from build123d import *

# Parameters (mm, degrees)
SKETCH1_R               = 10
BOSS_EXTRUDE1_DEPTH     = 15
BOSS_EXTRUDE2_START     = -2
BOSS_EXTRUDE2_OUTLINE_R = 1
BOSS_EXTRUDE2_DEPTH     = 2
SKETCH3_W               = 10
SKETCH3_H               = 3
BOSS_EXTRUDE3_DEPTH     = 2
SKETCH4_W               = 9.5
SKETCH4_H               = 2.5
SKETCH4_R               = 0.25
CUT_EXTRUDE1_DEPTH      = 3
SKETCH5_R               = 1.5
CUT_EXTRUDE2_DEPTH      = 3


# Read off the part's stored shape, not the designer's step: Boss-Extrude2
with BuildPart() as part:
    # Sketch1 → Boss-Extrude1 (new body)
    with BuildSketch(Plane.XY):
        Circle(SKETCH1_R)
    extrude(amount=BOSS_EXTRUDE1_DEPTH)

    # Boss-Extrude2 outline → Boss-Extrude2 (add)
    # profile 1 of 2: a face of its own
    with BuildSketch(Plane(origin=(0, 0, 0), x_dir=(-1, 0, 0), z_dir=(0, 0, -1)).offset(BOSS_EXTRUDE2_START)):
        with BuildLine():
            Line((5.599999975, -8.284926088), (14.179999754, -2.485477473))
            ThreePointArc((14.179999754, -2.485477473), (15.499999574, 0), (14.179999754, 2.485477473))
            Line((14.179999754, 2.485477473), (5.599999975, 8.284926088))
            ThreePointArc((5.599999975, 8.284926088), (10, 0), (5.599999975, -8.284926088))
        make_face()
        with Locations((12.5, 0)):
            Circle(BOSS_EXTRUDE2_OUTLINE_R, mode=Mode.SUBTRACT)
    # profile 2 of 2: a face of its own
    with BuildSketch(Plane(origin=(0, 0, 0), x_dir=(-1, 0, 0), z_dir=(0, 0, -1)).offset(BOSS_EXTRUDE2_START)):
        with BuildLine():
            Line((-14.179999754, -2.485477473), (-5.599999975, -8.284926088))
            ThreePointArc((-5.599999975, -8.284926088), (-10, 0), (-5.599999975, 8.284926088))
            Line((-5.599999975, 8.284926088), (-14.179999754, 2.485477473))
            ThreePointArc((-14.179999754, 2.485477473), (-15.499999574, 0), (-14.179999754, -2.485477473))
        make_face()
        with Locations((-12.5, 0)):
            Circle(BOSS_EXTRUDE2_OUTLINE_R, mode=Mode.SUBTRACT)
    extrude(amount=BOSS_EXTRUDE2_DEPTH)

    # Sketch3 → Boss-Extrude3 (add)
    with BuildSketch(Plane(origin=(0, 10, 0), x_dir=(1, 0, 0), z_dir=(0, 1, 0))):
        with Locations((0, -1.5)):
            Rectangle(SKETCH3_W, SKETCH3_H)
    extrude(amount=-BOSS_EXTRUDE3_DEPTH)

    # Sketch4 → Cut-Extrude1 (cut)
    with BuildSketch(Plane(origin=(0, 10, 0), x_dir=(1, 0, 0), z_dir=(0, 1, 0))):
        with Locations((0, -1.5)):
            Rectangle(SKETCH4_W, SKETCH4_H)
        with Locations(Location((-3, -1.5, 0), (0, 0, 270))):
            Circle(SKETCH4_R, mode=Mode.SUBTRACT)
        with Locations(Location((-1, -1.5, 0), (0, 0, 270))):
            Circle(SKETCH4_R, mode=Mode.SUBTRACT)
        with Locations(Location((1, -1.5, 0), (0, 0, 270))):
            Circle(SKETCH4_R, mode=Mode.SUBTRACT)
        with Locations(Location((3, -1.5, 0), (0, 0, 270))):
            Circle(SKETCH4_R, mode=Mode.SUBTRACT)
    extrude(amount=-CUT_EXTRUDE1_DEPTH, mode=Mode.SUBTRACT)

    # Sketch5 → Cut-Extrude2 (cut)
    with BuildSketch(Plane.XY.offset(15)):
        Circle(SKETCH5_R)
    extrude(amount=-CUT_EXTRUDE2_DEPTH, mode=Mode.SUBTRACT)


solid = part.part
Check sheet for the modelled part. Datum: model origin and axes. Units: mm. A direction names the side the tool comes from. Round coordinates to 2 decimals unless told otherwise and drop trailing zeros. Order: outer loops, then holes, each group sorted by start corner. A loop starts at its lowest first (then second) coordinate and runs counter-clockwise, first axis right, second up.
(1) Cross-section at D-D, the plane x = -13. Enter the section's corners in (y, z), and give its area (3 significant figures).
(2) Access from +Z, -Z, +X, -X, +Y, -Y to the whole of each face (thin tool, end or side, straight path). Record for faces 1 (the flat face through (5, 9, 2)), 2 (the flat face through (3.8, 9.6, 3)), 3 (the flat face through (0, 9, 2.75)), 4 (the cylindrical face through (-1.5, 0.07, 13.52)), 5 (the flat face through (-5, 9, 2)).
(3) Cross-section at C-C, the plane y = -3.5. Enter the section's corners in (x, z).
(4) Cross-section at A-A, the plane x = 12.5. Enter the section's corners in (y, z), and give its area (3 significant figures).
(5) Go/stop test with flat-tipped pins: P1, Ø0.9, axis at x = -0.5, y = -0.5, coming from the +Z side; P2, Ø1.5, axis at y = 9, z = 1, coming from the +X side; P3, Ø0.8, axis at x = 2.5, z = 2, coming from the +Y side. Record where each tip stops, or that it passes through.
(6) Scan lines: probe 1 along Y at (x, z) = (12.5, 0.9); probe 2 along Z at (x, y) = (10, 5); probe 3 along X at (y, z) = (-0.5, 12.5). Record each from-to range of solid material in increasing order.
(7) Cross-section at B-B, the plane y = 0. Enter the section's corners in (x, z), and give its area (3 significant figures).
(8) Draft check along Z on faces 6 (the cylindrical face through (4.614, -8.872, 7.395)), 7 (the flat face through (-11, -1, 2)), 8 (the flat face through (4.75, 9, 2)). Enter one of: pulls with the +Z half, pulls with the -Z half, needs draft (parallel to the pull), parting line crosses it, or undercut.
Check sheet entries:
1. outline: (-3.28, 0) - (-0.87, 0) - (-0.87, 2) - (-3.28, 2) - close; (0.87, 0) - (3.28, 0) - (3.28, 2) - (0.87, 2) - close
1. area: 9.67 mm2
2. face 1: +Z, -Z, +X, +Y
2. face 2: +Z, +X, +Y
2. face 3: +Y
2. face 4: +Z
2. face 5: +Z, -Z, -X, +Y
3. outline: (-12.68, 0) - (12.68, 0) - (12.68, 2) - (9.37, 2) - (9.37, 15) - (-9.37, 15) - (-9.37, 2) - (-12.68, 2) - close
4. outline: (-3.62, 0) - (-1, 0) - (-1, 2) - (-3.62, 2) - close; (1, 0) - (3.62, 0) - (3.62, 2) - (1, 2) - close
4. area: 10.5 mm2
5. P1: stops at z = 12
5. P2: stops at x = 5.65
5. P3: stops at y = 7
6. probe 1: y = -3.62 to -1, 1 to 3.62
6. probe 2: z = 0 to 2
6. probe 3: x = -9.99 to -1.41, 1.41 to 9.99
7. outline: (-15.5, 0) - (-13.5, 0) - (-13.5, 2) - (-15.5, 2) - close; (-11.5, 0) - (11.5, 0) - (11.5, 2) - (10, 2) - (10, 15) - (1.5, 15) - (1.5, 12) - (-1.5, 12) - (-1.5, 15) - (-10, 15) - (-10, 2) - (-11.5, 2) - close; (13.5, 0) - (15.5, 0) - (15.5, 2) - (13.5, 2) - close
7. area: 305 mm2
8. face 6: needs draft
8. face 7: pulls with the +Z half
8. face 8: undercut
